Verification items for the finished model (mm, model axes). Face numbers are marked on the shaded views. Give positions to 0.01 mm unless a question says otherwise; leave off trailing zeros. Write each loop counter-clockwise with the first axis right and the second up, starting at its lowest first coordinate (ties: lowest second). Pieces come first, ordered by that corner, then holes. Notation, with made-up numbers: (-25, 62.25) -> (-20, 62.25) arc R18 cw to (-20, 73.25) -> close; hole circle Ø1 at (31.25, 78). An arc over 180 degrees is marked (long way). Use CSV: the item, a comma, the result in double quotes. Start each with the question number.
```python
from build123d import *

# Parameters (mm, degrees)
BOSS_EXTRUDE1_DEPTH = 1.6
SKETCH3_W           = 2.15
SKETCH3_H           = 30
SKETCH4_W           = 2.15
SKETCH4_H           = 30
SKETCH5_R           = 1.5
CUT_EXTRUDE1_DEPTH  = 28


with BuildPart() as part:
    # Sketch2 → Boss-Extrude1 (new body)
    with BuildSketch(Plane.XY):
        with BuildLine():
            Line((-20.5, -0.8), (-13.5, -0.8))
            ThreePointArc((-13.5, -0.8), (-12.227207794, -0.272792206), (-11.7, 1))
            Line((-11.7, 1), (-11.7, 7))
            ThreePointArc((-11.7, 7), (-11, 7.7), (-10.3, 7))
            Line((-10.3, 7), (-10.3, 0))
            Line((-10.3, 0), (-10.3, -7))
            ThreePointArc((-10.3, -7), (-8, -9.3), (-5.7, -7))
            Line((-5.7, -7), (-5.7, 0))
            Line((-5.7, 0), (-5.7, 7))
            ThreePointArc((-5.7, 7), (-5, 7.7), (-4.3, 7))
            Line((-4.3, 7), (-4.3, 0))
            Line((-4.3, 0), (-4.3, -7))
            ThreePointArc((-4.3, -7), (-2, -9.3), (0.3, -7))
            Line((0.3, -7), (0.3, 0))
            Line((0.3, 0), (0.3, 7))
            ThreePointArc((0.3, 7), (1, 7.7), (1.7, 7))
            Line((1.7, 7), (1.7, 0))
            Line((1.7, 0), (1.7, -7))
            ThreePointArc((1.7, -7), (4, -9.3), (6.3, -7))
            Line((6.3, -7), (6.3, -1))
            ThreePointArc((6.3, -1), (6.358578644, -0.858578644), (6.5, -0.8))
            Line((6.5, -0.8), (13.5, -0.8))
            ThreePointArc((13.5, -0.8), (14.3, 0), (13.5, 0.8))
            Line((13.5, 0.8), (6.5, 0.8))
            ThreePointArc((6.5, 0.8), (5.227207794, 0.272792206), (4.7, -1))
            Line((4.7, -1), (4.7, -7))
            ThreePointArc((4.7, -7), (4, -7.7), (3.3, -7))
            Line((3.3, -7), (3.3, 0))
            Line((3.3, 0), (3.3, 7))
            ThreePointArc((3.3, 7), (1, 9.3), (-1.3, 7))
            Line((-1.3, 7), (-1.3, 0))
            Line((-1.3, 0), (-1.3, -7))
            ThreePointArc((-1.3, -7), (-2, -7.7), (-2.7, -7))
            Line((-2.7, -7), (-2.7, 0))
            Line((-2.7, 0), (-2.7, 7))
            ThreePointArc((-2.7, 7), (-5, 9.3), (-7.3, 7))
            Line((-7.3, 7), (-7.3, 0))
            Line((-7.3, 0), (-7.3, -7))
            ThreePointArc((-7.3, -7), (-8, -7.7), (-8.7, -7))
            Line((-8.7, -7), (-8.7, 0))
            Line((-8.7, 0), (-8.7, 7))
            ThreePointArc((-8.7, 7), (-11, 9.3), (-13.3, 7))
            Line((-13.3, 7), (-13.3, 1))
            ThreePointArc((-13.3, 1), (-13.358578644, 0.858578644), (-13.5, 0.8))
            Line((-13.5, 0.8), (-20.5, 0.8))
            ThreePointArc((-20.5, 0.8), (-21.3, 0), (-20.5, -0.8))
        make_face()
    extrude(amount=BOSS_EXTRUDE1_DEPTH)

    # Sketch3 → Revolve1 (revolve)
    with BuildSketch(Plane(origin=(0, 0, 0), x_dir=(1, 0, 0), z_dir=(0, 1, 0)), mode=Mode.PRIVATE) as revolve1_sk:
        with Locations((-21.575, 13.4)):
            Rectangle(SKETCH3_W, SKETCH3_H)
    revolve(revolve1_sk.sketch.rotate(Axis((-20.5, 0, 1.6), (0, 0, -1)), 180), axis=Axis((-20.5, 0, 1.6), (0, 0, -1)))

    # Sketch4 → Revolve2 (revolve)
    with BuildSketch(Plane(origin=(0, 0, 0), x_dir=(1, 0, 0), z_dir=(0, 1, 0))):
        with Locations((14.575, 13.4)):
            Rectangle(SKETCH4_W, SKETCH4_H)
    revolve(axis=Axis((13.5, 0, 1.6), (0, 0, -1)))

    # Sketch5 → Cut-Extrude1 (cut)
    with BuildSketch(Plane(origin=(0, 0, -28.4), x_dir=(-1, 0, 0), z_dir=(0, 0, -1))):
        with Locations((20.5, 0)):
            Circle(SKETCH5_R)
        with Locations((-13.5, 0)):
            Circle(SKETCH5_R)
    extrude(amount=-CUT_EXTRUDE1_DEPTH, mode=Mode.SUBTRACT)


solid = part.part
```
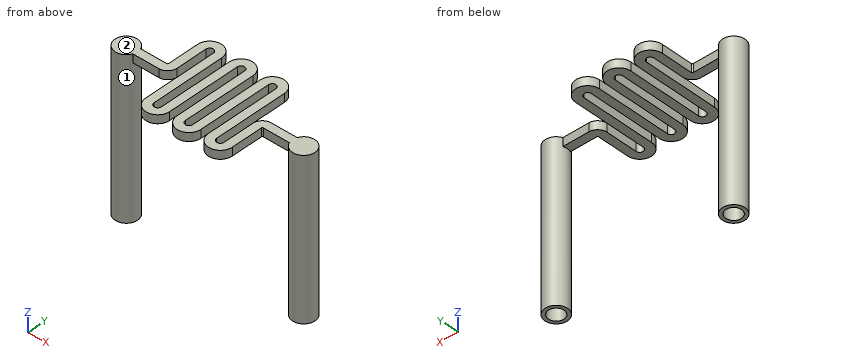
(1) Section check B-B on z = -9.25. Record the cut outline in (x, y), then the cut area to 3 significant figures.
(2) Thickness scan on line 1 (Y direction, x = 13.5, z = -20.25); line 2 (Z direction, x = -15, y = -0.25); line 3 (Y direction, x = -20, z = -17.5). Record the ranges inside material, lowest first. Write a range as from..to.
(3) Draft check along X on the marked faces 1 and 2. Enter one of: released by +X, released by -X, zero draft, split by the parting line, or undercut.
(4) Go/stop test with flat-tipped pins: pin 1 (0.5 mm diameter, centred on x = 8, z = 0.5, fed in from -Y); pin 2 (0.8 mm diameter, centred on y = -2, z = 0.5, fed in from -X); pin 3 (0.5 mm diameter, centred on y = -2, z = 1, fed in from +X). Record where each tip stops, or that it passes through.
(5) Section check A-A on y = -4.5. Record the cut outline in (x, z).
(6) Section check D-D on y = 0. Give the number of separate pieces and of enclosed holes in the cut face, then the cut area to 3 significant figures.
(7) Section check C-C on x = 13.5. Record the cut outline in (y, z).
Data:
1,outline,"circle Ø4.3 at (-20.5, 0); circle Ø4.3 at (13.5, 0); hole circle Ø3 at (-20.5, 0); hole circle Ø3 at (13.5, 0)"
1,area,"14.9 mm2"
2,line 1,"y = -2.15..-1.5, 1.5..2.15"
2,line 2,"z = 0..1.6"
2,line 3,"y = -2.09..-1.41, 1.41..2.09"
3,face 1,"undercut"
3,face 2,"zero draft"
4,pin 1,"stops at y = -0.8"
4,pin 2,"stops at x = -21.94"
4,pin 3,"stops at x = 14.75"
5,outline,"(-10.3, 0) -> (-8.7, 0) -> (-8.7, 1.6) -> (-10.3, 1.6) -> close; (-7.3, 0) -> (-5.7, 0) -> (-5.7, 1.6) -> (-7.3, 1.6) -> close; (-4.3, 0) -> (-2.7, 0) -> (-2.7, 1.6) -> (-4.3, 1.6) -> close; (-1.3, 0) -> (0.3, 0) -> (0.3, 1.6) -> (-1.3, 1.6) -> close; (1.7, 0) -> (3.3, 0) -> (3.3, 1.6) -> (1.7, 1.6) -> close; (4.7, 0) -> (6.3, 0) -> (6.3, 1.6) -> (4.7, 1.6) -> close"
6,separate pieces,"7"
6,enclosed holes,"0"
6,area,"123 mm2"
7,outline,"(-2.15, -28.4) -> (-1.5, -28.4) -> (-1.5, -0.4) -> (1.5, -0.4) -> (1.5, -28.4) -> (2.15, -28.4) -> (2.15, 1.6) -> (-2.15, 1.6) -> close"
